Autodesk Inventor part; units mm, degrees
ref_plane "YZ Plane" through (0, 0, 0) normal (1, 0, 0) x (0, 1, 0)
ref_plane "XZ Plane" through (0, 0, 0) normal (0, 1, 0) x (-1, 0, 0)
ref_plane "XY Plane" through (0, 0, 0) normal (0, 0, 1) x (1, 0, 0)
ref_plane "Work Plane1" through (67.8466, -36.9116, -13.6178) normal (0, 0, -1) x (1, 0, 0)
sketch "Sketch1" plane through (67.8466, -36.9116, -13.6178) normal (0, 0, -1) x (1, 0, 0)
  circle A0 centre (-25.3126, -0.0255) radius 25
  circle A1 centre (-25.3126, -0.0255) radius 25.15
  circle A2 centre (-25.3126, -0.0255) radius 27.15
  point P0 (-67.8466, -36.9116)
  dimension "d8" = 0.15
  dimension "d9" = 2
  dimension "d26" = 54.3
extrude "Extrusion2" add sketch "Sketch1" along normal mid plane 20 contours A2
fillet "Fillet3" radius 2 1 edges at (15.384, -36.8861, -3.6178)
ref_plane "Work Plane3" through (73.8334, -36.8861, -23.6178) normal (0, 1, 0) x (-1, 0, 0)
sketch "Sketch4" plane through (73.8334, -36.8861, -23.6178) normal (0, 1, 0) x (-1, 0, 0)
  line L0 (6.1494, 20) -> (6.1494, 0) construction
  line L1 (56.4494, 20) -> (56.4494, 0) construction
  line L2 (4.1494, 0) -> (6.1494, -2)
  line L3 (6.1494, -2) -> (6.1494, -4)
  line L4 (6.1494, -4) -> (8.1494, -4)
  line L5 (31.2994, 0.6713) -> (31.2994, 28.2514) construction
  line L6 (31.2994, 28.2514) -> (31.2994, -7.4559) construction
  line L7 (8.1494, -0.2025) -> (6.2913, -0.2025)
  line L8 (4.1494, 0) -> (6.1496, 0)
  line L9 (4.1494, 0) -> (6.1494, 0) construction
  line L10 (6.2911, 0) -> (6.9778, 0) construction
  line L11 (6.2913, -0.2025) -> (6.1496, -0.2025)
  line L12 (6.1496, -0.2025) -> (6.1496, 0)
  line L13 (8.2994, -0.2025) -> (8.2994, 19.7975) construction
  line L14 (8.1494, -0.2025) -> (8.2994, -0.2025)
  line L15 (8.2994, -0.2025) -> (8.2994, -4)
  line L16 (8.2994, -4) -> (8.1494, -4)
  point P0 (73.8334, 23.6178)
  dimension "d18" = 2
revolve "Revolution1" add sketch "Sketch4" angle 360 about axis through (42.534, -36.8861, 4.6336) along (0, 0, -1)
fillet "Fillet5" radius 2 2 edges at (17.384, -36.8861, -25.6178) (15.384, -36.8861, -23.6178)
ref_plane "Work Plane12" through (42.534, -36.8861, -15.6178) normal (0, 0, -1) x (0, 1, 0)
sketch "Sketch6" plane through (42.534, -36.8861, -15.6178) normal (0, 0, -1) x (0, 1, 0)
  line L0 (5, 31.75) -> (-5, 31.75)
  line L1 (31.75, -7.9821) -> (31.75, 7.9821)
  line L2 (7.9821, 31.75) -> (-7.9821, 31.75)
  line L3 (-31.75, 7.9821) -> (-31.75, -7.9821)
  line L4 (-7.9821, -31.75) -> (7.9821, -31.75)
  arc A0 (-31.75, -7.9821) -> (-7.9821, -31.75) centre (0, 0) ccw
  arc A1 (-7.9821, 31.75) -> (-31.75, 7.9821) centre (0, 0) ccw
  arc A2 (7.9821, -31.75) -> (31.75, -7.9821) centre (0, 0) ccw
  arc A3 (31.75, 7.9821) -> (7.9821, 31.75) centre (0, 0) ccw
  line L5 (-1.7661, -31.75) -> (7.9821, -31.75)
  arc A4 (-7.9821, 31.75) -> (-31.75, 7.9821) centre (0, 0) ccw
  arc A5 (-31.75, -7.9821) -> (-7.9821, -31.75) centre (0, 0) ccw
  arc A6 (7.9821, -31.75) -> (31.75, -7.9821) centre (0, 0) ccw
  arc A7 (31.75, 7.9821) -> (7.9821, 31.75) centre (0, 0) ccw
extrude "Extrusion4" add sketch "Sketch6" along normal blind 2
sketch "Sketch7" plane through (42.534, -36.8861, -27.6178) normal (0, 0, -1) x (-1, 0, 0)
  circle A0 centre (0, 0) radius 23 construction
  circle A1 centre (0, 0) radius 25.15 construction
  line L0 (0, -40.051) -> (0, 42.9038) construction
  line L1 (-48.7042, 0) -> (50.8727, 0) construction
ref_plane "plano de separación con el cono" through (42.534, -36.8861, -28.0178) normal (0, 0, -1) x (-1, 0, 0)
sketch "Sketch8" plane through (42.534, -36.8861, -15.6178) normal (0, 0, 1) x (1, 0, 0)
  circle A0 centre (0, 0) radius 25.15
  point P0 (-42.534, 36.8861)
extrude "Extrusion5" cut sketch "Sketch8" against normal up to surface (2 mm away)
equation "\"d8\" = HOLE_TOLERANCE"
equation "\"HOLE_TOLERANCE\" = 0.15"
properties part number "adaptador_cono" material "PET Plastic"
For this review, take the finished solid that the model builds, in its own axes (mm). A direction names the side the tool comes from. Round coordinates to 2 decimals unless told otherwise and drop trailing zeros. Write each loop counter-clockwise with the first axis right and the second up, starting at its lowest first coordinate (ties: lowest second). Pieces come first, ordered by that corner, then holes. Notation, with made-up numbers: M -30.5,-14 L 17.5,-14 A34 cw 17.5,25 Z; hole C 15.5,-7.75 d1. An arc over 180 degrees is marked long. Write item = value, one per line. Start each with the question number.
(1) We need section A-A (z = -10.25). Give the boundary of the cut face in (x, y).
(2) The part is to be moulded in two halves that separate along X. For faces 4 (the face through (19.21, -59.86, -16.6)), 5 (the face through (42, -5.136, -17)), 6 (the face through (37.548, -14.433, -25.746)), say which applies: +X half, -X half, draft (parallel to the pull), parting line (faces both ways), or undercut.
(3) We need section B-B (x = 70.5). Give the boundary of the cut face in (y, z).
(4) For line 1 along Z through (x, y) = (63, -50.5); line 2 along X through (y, z) = (-53.5, -26.5); line 3 along Y through (x, z) = (33.5, -5.25), list the stretches that pass through material, from the lowest coordinate up.
(5) For faces 1 (the face through (53.6, -16.5, -23.82)), 2 (the face through (68.43, -45.04, -20.24)), 3 (the face through (43, -68.636, -17)), list the 3-axis set-ups (+Z, -Z, +X, -X, +Y, -Y) from which the entire face can be reached by the end or side of a thin tool; tool diameter is ignored.
(6) Clearance check with flat-ended pins moving along their axes: pin 1 Ø12 at (y, z) = (-41.5, -22.5) entering from +X; pin 2 Ø4 at (x, y) = (59.5, -46) entering from -Z; pin 3 Ø1.5 at (x, z) = (67.5, -19) entering from -Y; pin 4 Ø12 at (y, z) = (-17, -11) entering from +X. State where each tip first meets the part, or that it passes through.
Results found:
q1.outline = C 42.53,-36.89 d54.3; hole C 42.53,-36.89 d50.3
q2.face_4 = -X half
q2.face_5 = draft
q2.face_6 = undercut
q3.outline = M -53.91,-17.62 L -19.87,-17.62 L -19.87,-15.62 L -53.91,-15.62 Z
q4.line_1 = -27.62 to -23.82
q4.line_2 = 23.65 to 26.63, 58.44 to 61.42
q4.line_3 = -62.45 to -60.36, -13.41 to -11.32
q5.face_1 = +Z
q5.face_2 = -Z
q5.face_3 = +Z, -Z, +X, -X, -Y
q6.pin_1 = 74.28
q6.pin_2 = through
q6.pin_3 = -49.16
q6.pin_4 = 71.06
